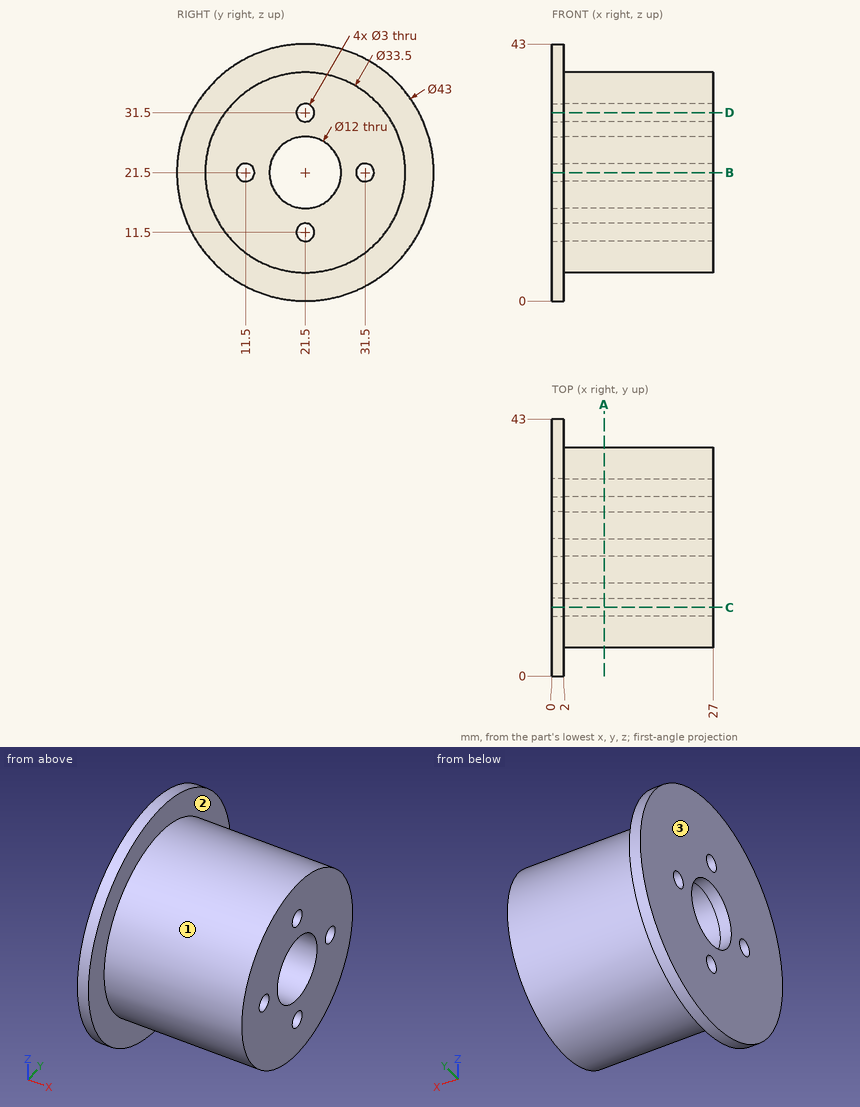
Input: dimensioned drawing with shaded views. Units: mm. Origin: part minimum x, y, z. Round coordinates to 2 decimals unless told otherwise and drop trailing zeros. Loops run counter-clockwise (first coordinate to the right, second up) from the corner with the lowest first, then second, coordinate; pieces in that order, holes last. Notation, with made-up numbers: (3, 35.25) -> (35, 35.25) arc R4 cw to (35, 42.25) -> close; hole circle Ø1 at (25.25, 29). An arc over 180 degrees is marked (long way). Answer as a JSON object with one key per item and string values. Group by question number.
1) Draft query along X for the marked faces 1, 2 and 3. Return one class per face: +X half, -X half, draft (parallel to the pull), parting line (faces both ways), or undercut.
2) Pin query (flat end, axial travel): pin 1 (8 mm diameter, centred on x = 8.5, z = 28.5, fed in from +Y); pin 2 (3 mm diameter, centred on x = 20.5, y = 29, fed in from +Z); pin 3 (1.8 mm diameter, centred on y = 11.5, z = 21.5, fed in from -X); pin 4 (10 mm diameter, centred on x = 8, y = 17.5, fed in from +Z). Return the tip coordinate at first contact, or that it passes through.
3) Section query C-C on y = 11.5. Output: boundary loops of the cut face in (x, z).
4) Section query B-B on z = 21.5. Output: boundary loops of the cut face in (x, y).
5) Section query A-A on x = 8.75. Output: boundary loops of the cut face in (y, z).
6) Ray query, L1, parallel to Z at x = 13.5, y = 21.5; L2, parallel to X at y = 22, z = 3.5; L3, parallel to Z at x = 7, y = 18.5. Return the intervals inside material, ascending.
Reply:
{
 "1": {"face 1": "draft", "face 2": "+X half", "face 3": "-X half"},
 "2": {"pin 1": "stops at y = 37.98", "pin 2": "stops at z = 37.14", "pin 3": "passes through", "pin 4": "stops at z = 38.25"},
 "3": {"outline": "(0, 2.47) -> (2, 2.47) -> (2, 8.06) -> (27, 8.06) -> (27, 20) -> (0, 20) -> close; (0, 23) -> (27, 23) -> (27, 34.94) -> (2, 34.94) -> (2, 40.53) -> (0, 40.53) -> close"},
 "4": {"outline": "(0, 0) -> (2, 0) -> (2, 4.75) -> (27, 4.75) -> (27, 10) -> (0, 10) -> close; (0, 13) -> (27, 13) -> (27, 15.5) -> (0, 15.5) -> close; (0, 27.5) -> (27, 27.5) -> (27, 30) -> (0, 30) -> close; (0, 33) -> (27, 33) -> (27, 38.25) -> (2, 38.25) -> (2, 43) -> (0, 43) -> close"},
 "5": {"outline": "circle Ø33.5 at (21.5, 21.5); hole circle Ø3 at (11.5, 21.5); hole circle Ø12 at (21.5, 21.5); hole circle Ø3 at (21.5, 11.5); hole circle Ø3 at (21.5, 31.5); hole circle Ø3 at (31.5, 21.5)"},
 "6": {"L1": "z = 4.75 to 10, 13 to 15.5, 27.5 to 30, 33 to 38.25", "L2": "x = 0 to 2", "L3": "z = 5.02 to 16.3, 26.7 to 37.98"}
}
